Could you check a few things on this model? Use its own coordinates, in mm. A direction names the side the tool comes from. Round coordinates to 2 decimals unless told otherwise and drop trailing zeros. Loops run counter-clockwise (first coordinate to the right, second up) from the corner with the lowest first, then second, coordinate; pieces in that order, holes last. Notation, with made-up numbers: (4, 45.5) -> (30, 45.5) arc R22 cw to (30, 71.5) -> close; hole circle Ø5 at (-39, 23.25). An arc over 180 degrees is marked (long way). One line per item, written item: value.
```python
from build123d import *

# Parameters (mm, degrees)
PAD_DEPTH     = 10
SKETCH001_R   = 8
SKETCH001_R_2 = 14
SKETCH001_R_3 = 1.8
POCKET_DEPTH  = 10.001


with BuildPart() as part:
    # Sketch → Pad (new body)
    with BuildSketch(Plane.XY):
        Polygon((0, 0), (560, 0), (570, 0), (570, 50), (560, 50), (560, 135.6), (570, 135.6), (570, 185.6), (560, 185.6), (0, 185.6), (-10, 185.6), (-10, 135.6), (0, 135.6), (0, 50), (-10, 50), (-10, 0), align=None)
    extrude(amount=PAD_DEPTH)

    # Sketch001 → Pocket (cut, through all)
    with BuildSketch(Plane.XY.offset(10)):
        with Locations((70, 74.24)):
            Circle(SKETCH001_R)
        with Locations((135, 102.76)):
            Circle(SKETCH001_R_2)
        with Locations((180, 125.26)):
            Circle(SKETCH001_R_2)
        with Locations((225, 125.26)):
            Circle(SKETCH001_R_2)
        with Locations((135, 57.76)):
            Circle(SKETCH001_R_2)
        with Locations((180, 80.26)):
            Circle(SKETCH001_R_2)
        with Locations((225, 80.26)):
            Circle(SKETCH001_R_2)
        with Locations((350, 74.24)):
            Circle(SKETCH001_R)
        with Locations((415, 102.76)):
            Circle(SKETCH001_R_2)
        with Locations((460, 125.26)):
            Circle(SKETCH001_R_2)
        with Locations((505, 125.26)):
            Circle(SKETCH001_R_2)
        with Locations((505, 80.26)):
            Circle(SKETCH001_R_2)
        with Locations((460, 80.26)):
            Circle(SKETCH001_R_2)
        with Locations((415, 57.76)):
            Circle(SKETCH001_R_2)
        with Locations((50, 116.74)):
            Circle(SKETCH001_R_3)
        with Locations((90, 116.74)):
            Circle(SKETCH001_R_3)
        with Locations((50, 31.74)):
            Circle(SKETCH001_R_3)
        with Locations((90, 31.74)):
            Circle(SKETCH001_R_3)
        with Locations((330, 116.74)):
            Circle(SKETCH001_R_3)
        with Locations((370, 116.74)):
            Circle(SKETCH001_R_3)
        with Locations((370, 31.74)):
            Circle(SKETCH001_R_3)
        with Locations((330, 31.74)):
            Circle(SKETCH001_R_3)
    extrude(amount=-POCKET_DEPTH, mode=Mode.SUBTRACT)


solid = part.part
```
(1) Imagine slicing it at B-B on x = 505. Write out the boundary of the cut face in (y, z), then the cut area to 3 significant figures.
Results below:
outline: (0, 0) -> (66.26, 0) -> (66.26, 10) -> (0, 10) -> close; (94.26, 0) -> (111.26, 0) -> (111.26, 10) -> (94.26, 10) -> close; (139.26, 0) -> (185.6, 0) -> (185.6, 10) -> (139.26, 10) -> close
area: 1,300 mm²
(2) Imagine slicing it at A-A on x = 350. Write out the boundary of the cut face in (y, z), then the cut area to 3 significant figures.
Results below:
outline: (0, 0) -> (66.24, 0) -> (66.24, 10) -> (0, 10) -> close; (82.24, 0) -> (185.6, 0) -> (185.6, 10) -> (82.24, 10) -> close
area: 1,700 mm²
(3) We'd pull the mould along X, two halves only. Please class faces 4 (the face through (518.35, 84.47, 5.07)), 5 (the face through (0, 93, 5)), 6 (the face through (565, 135.6, 5)): +X half, -X half, draft (parallel to the pull), parting line (faces both ways), or undercut.
Results below:
face 4: undercut
face 5: -X half
face 6: draft
(4) Imagine slicing it at D-D on z = 6. Give the number of separate pieces and of enclosed holes in the cut face, then the cut area to 3 significant figures.
Results below:
separate pieces: 1
enclosed holes: 22
area: 98,100 mm²
(5) Imagine slicing it at C-C on y = 57.76. Write out the boundary of the cut face in (x, z), then the cut area to 3 significant figures.
Results below:
outline: (0, 0) -> (121, 0) -> (121, 10) -> (0, 10) -> close; (149, 0) -> (401, 0) -> (401, 10) -> (149, 10) -> close; (429, 0) -> (560, 0) -> (560, 10) -> (429, 10) -> close
area: 5,040 mm²
(6) Please list where these lines run through material, in increasing order: L1, parallel to Y at x = 50, z = 7; L2, parallel to Y at x = 505, z = 4.75; L3, parallel to X at y = 129.5, z = 9.
Results below:
L1: y = 0 to 29.94, 33.54 to 114.94, 118.54 to 185.6
L2: y = 0 to 66.26, 94.26 to 111.26, 139.26 to 185.6
L3: x = 0 to 166.66, 193.34 to 211.66, 238.34 to 446.66, 473.34 to 491.66, 518.34 to 560
(7) On a 3-axis mill with a long thin cutter (end or side, diameter ignored), from which of +Z, -Z, +X, -X, +Y, -Y can I reach the whole of each face in a straight line? I mean faces 1 (the face through (560, 92, 5)), 2 (the face through (-5, 50, 5)), 3 (the face through (276, 0, 5)). Say none if no direction works.
Results below:
face 1: +Z, -Z, +X
face 2: +Z, -Z, -X
face 3: +Z, -Z, +X, -X, -Y
(8) For pin 1 Ø4 at (x, y) = (90, 116.74) entering from +Z; pin 2 Ø3 at (y, z) = (87, 6.5) entering from +X, each with a flat end and sliding along its axis, tell me the tip position at first contact or that it passes through.
Results below:
pin 1: stops at z = 10
pin 2: stops at x = 560
